from build123d import *

# Parameters (mm, degrees)
ESQUISSE1_W         = 200
ESQUISSE1_H         = 28.284
BOSS_EXTRU_3_DEPTH  = 8
CHANFREIN1_SIZE     = 20
ESQUISSE4_R         = 2
CUT_EXTRUDE5_DEPTH  = 30
FILLET1_R           = 8
SKETCH2_R           = 1.5
SKETCH2_R_2         = 3.75
CUT_EXTRUDE1_DEPTH  = 8
FILLET9_R           = 1
FILLET10_R          = 1
SKETCH6_W           = 138
SKETCH6_H           = 28.284
BOSS_EXTRUDE3_DEPTH = 12
CHAMFER2_SIZE       = 10
CHAMFER2_SIZE2      = 27.474774195
CUT_EXTRUDE6_DEPTH  = 20
CHAMFER8_SIZE       = 10
CHAMFER9_SIZE       = 10


# Some blends are built 0.0001 mm under size
with BuildPart() as part:
    # Esquisse1 → Boss.-Extru.3 (new body)
    with BuildSketch(Plane.XY):
        with Locations((100, 14.142)):
            Rectangle(ESQUISSE1_W, ESQUISSE1_H)
    extrude(amount=BOSS_EXTRU_3_DEPTH)

    # Chanfrein1
    # the kernel refuses this chamfer: 20 mm, written as the material it takes off along each edge
    with BuildSketch(Plane(origin=(200, -51.433659759, 8), x_dir=(0.027495876610586317, 0, -0.9996219169112968), z_dir=(0, 1, 0))) as chanfrein1_piece_1:
        Polygon((CHANFREIN1_SIZE * 0.999621916911, CHANFREIN1_SIZE * 0.0274958766106), (-CHANFREIN1_SIZE * 0.0274958766106, CHANFREIN1_SIZE * 0.999621916911), (0, 0), align=None)
    extrude(amount=131.151319519, mode=Mode.SUBTRACT)

    # Esquisse4 → Cut-Extrude5 (cut)
    with BuildSketch(Plane.XY.offset(8)):
        with Locations((176, 7.142)):
            Circle(ESQUISSE4_R)
        with Locations((176, 21.142)):
            Circle(ESQUISSE4_R)
    extrude(amount=-CUT_EXTRUDE5_DEPTH, mode=Mode.SUBTRACT)

    # Fillet1
    fillet1_edges = [part.edges().sort_by_distance(p)[0] for p in [
        (0, 14.142, 0),
    ]]
    fillet(fillet1_edges, radius=FILLET1_R - 0.0001)  # a hair under: the kernel refuses the full size

    # Sketch2 → Cut-Extrude1 (cut)
    with BuildSketch(Plane.XY.offset(8)):
        with Locations((10.180485171, 7.281517741)):
            Circle(SKETCH2_R)
        with Locations((24.142857006, 20.883346587)):
            Circle(SKETCH2_R)
        with Locations((17.323003706, 13.918303783)):
            Circle(SKETCH2_R_2)
        Polygon((14.943517177, 18.243352736), (12.822196834, 16.122032392), (9.422196834, 19.522032392), (11.543517177, 21.643352736), align=None)
        Polygon((19.379761465, 9.564467761), (22.780003771, 6.164594852), (24.901208877, 8.286030428), (21.501081812, 11.685788108), align=None)
    extrude(amount=-CUT_EXTRUDE1_DEPTH, mode=Mode.SUBTRACT)

    # Fillet9
    fillet9_edges = [part.edges().sort_by_distance(p)[0] for p in [
        (9.422196834, 19.522032392, 4),
        (11.543517177, 21.643352736, 4),
        (14.943517177, 18.243352736, 4),
        (12.822196834, 16.122032392, 4),
    ]]
    fillet(fillet9_edges, radius=FILLET9_R)

    # Fillet10
    fillet10_edges = [part.edges().sort_by_distance(p)[0] for p in [
        (24.901208877, 8.286030428, 4),
        (22.780003771, 6.164594852, 4),
        (19.379761465, 9.564467761, 4),
        (21.501081812, 11.685788108, 4),
    ]]
    fillet(fillet10_edges, radius=FILLET10_R)

    # Sketch6 → Boss-Extrude3 (add)
    with BuildSketch(Plane(origin=(0, 0, 0), x_dir=(-1, 0, 0), z_dir=(0, 0, -1))):
        with Locations((-98.018199025, 14.142)):
            Rectangle(SKETCH6_W, SKETCH6_H)
    extrude(amount=BOSS_EXTRUDE3_DEPTH)

    # Chamfer2
    chamfer2_edges = [part.edges().sort_by_distance(p)[0] for p in [
        (29.018199025, 14.142, -12),
    ]]
    chamfer2_side = [part.faces().sort_by_distance(p)[0] for p in [
        (29.018199025, 14.142, -6),
    ]]
    chamfer(chamfer2_edges, length=CHAMFER2_SIZE, length2=CHAMFER2_SIZE2, reference=chamfer2_side[0])

    # Sketch4 → Cut-Extrude6 (cut)
    with BuildSketch(Plane.XY.offset(8)):
        Polygon((47.82891302, 12.144), (28, 12.144), (28, 2.144), (37.82891302, 2.144), align=None)
        Polygon((62.82891302, 2.144), (52.82891302, 12.144), (42.82891302, 2.144), align=None)
        Polygon((77.82891302, 12.144), (57.82891302, 12.144), (67.82891302, 2.144), align=None)
        Polygon((82.82891302, 12.144), (72.82891302, 2.144), (93.894603713, 2.144), align=None)
        Polygon((108.238219115, 12.144), (87.82891302, 12.144), (98.894603713, 2.144), align=None)
        Polygon((113.238219115, 12.144), (103.894603713, 2.144), (123.940714423, 2.144), align=None)
        Polygon((138.940714423, 12.144), (118.238219115, 12.144), (128.940714423, 2.144), align=None)
        Polygon((143.940714423, 12.144), (133.940714423, 2.144), (152.455696505, 2.144), align=None)
        Polygon((170, 12.144), (148.940714423, 12.144), (157.455696505, 2.144), (170, 2.144), align=None)
        Polygon((157.455696505, 26.144), (148.940714423, 16.144), (170, 16.144), (170, 26.144), align=None)
        Polygon((152.455696505, 26.144), (133.940714423, 26.144), (143.940714423, 16.144), align=None)
        Polygon((128.940714423, 26.144), (118.238219115, 16.144), (138.940714423, 16.144), align=None)
        Polygon((123.940714423, 26.144), (103.894603713, 26.144), (113.238219115, 16.144), align=None)
        Polygon((98.894603713, 26.144), (87.82891302, 16.144), (108.238219115, 16.144), align=None)
        Polygon((93.894603713, 26.144), (72.82891302, 26.144), (82.82891302, 16.144), align=None)
        Polygon((67.82891302, 26.144), (57.82891302, 16.144), (77.82891302, 16.144), align=None)
        Polygon((62.82891302, 26.144), (42.82891302, 26.144), (52.82891302, 16.144), align=None)
        Polygon((37.82891302, 26.144), (28, 26.144), (28, 16.144), (47.82891302, 16.144), align=None)
    extrude(amount=-CUT_EXTRUDE6_DEPTH, mode=Mode.SUBTRACT)

    # Chamfer8
    chamfer8_edges = [part.edges().sort_by_distance(p)[0] for p in [
        (167.018199025, 1.072, -12),
        (167.018199025, 14.144, -12),
    ]]
    chamfer(chamfer8_edges, length=CHAMFER8_SIZE)

    # Chamfer9
    chamfer9_edges = [part.edges().sort_by_distance(p)[0] for p in [
        (167.018199025, 27.214, -12),
    ]]
    chamfer(chamfer9_edges, length=CHAMFER9_SIZE)


solid = part.part
Source: CAD feature listing. Evaluate the final solid. Frame: model axes, mm. Round coordinates to 2 decimals unless told otherwise and drop trailing zeros. Loops run counter-clockwise (first coordinate to the right, second up) from the corner with the lowest first, then second, coordinate; pieces in that order, holes last. Notation, with made-up numbers: (10, 3.25) - (65, 3.25) arc R16 cw to (65, 30.25) - close; hole circle Ø7 at (-11, 19.5). An arc over 180 degrees is marked (long way). Write item = value, one per line. Start each with the question number.
Item 1: First-contact query: pin 1 Ø4 at (x, y) = (116, 25.5) entering from -Z; pin 2 Ø3.5 at (x, y) = (176, 7.142) entering from -Z; pin 3 Ø1.6 at (y, z) = (27, -1) entering from +X; pin 4 Ø1 at (y, z) = (1.5, -1.5) entering from -X. Flat tips, straight axial feed; report the tip coordinate or a pass-through.
Item 2: Section query B-B on x = 32. Output: boundary loops of the cut face in (y, z), plus the area to 3 significant figures.
Item 3: Mould query, pull axis Y, two halves, no side actions, for faces 1 (the face through (108.501, 21.214, -1.86)), 2 (the face through (38, 12.144, 2)), 3 (the face through (107, 14, -12)). Classes: released by +Y, released by -Y, zero draft, split by the parting line, or undercut.
Item 4: Material intervals for line 1 (Y direction, x = 176, z = 3); line 2 (Y direction, x = 163, z = -3); line 3 (Y direction, x = 76, z = -1), sorted ascending.
Item 5: Section query A-A on x = 176. Output: boundary loops of the cut face in (y, z), plus the area to 3 significant figures.
Results list:
q1.pin_1 = -12
q1.pin_2 = through
q1.pin_3 = 167.02
q1.pin_4 = 29.02
q2.outline = (0, -3.09) - (2.14, -3.09) - (2.14, 8) - (0, 8) - close; (12.14, -3.09) - (16.14, -3.09) - (16.14, 8) - (12.14, 8) - close; (26.14, -3.09) - (28.28, -3.09) - (28.28, 8) - (26.14, 8) - close
q2.area = 91.8 mm²
q3.face_1 = undercut
q3.face_2 = undercut
q3.face_3 = zero draft
q4.line_1 = 0 to 5.14, 9.14 to 19.14, 23.14 to 28.28
q4.line_2 = 0 to 2.14, 12.14 to 16.14, 26.14 to 28.28
q4.line_3 = 0 to 2.14, 5.32 to 10.32, 12.14 to 16.14, 17.97 to 22.97, 26.14 to 28.28
q5.outline = (0, 0) - (5.14, 0) - (5.14, 8) - (0, 8) - close; (9.14, 0) - (19.14, 0) - (19.14, 8) - (9.14, 8) - close; (23.14, 0) - (28.28, 0) - (28.28, 8) - (23.14, 8) - close
q5.area = 162 mm²
